Drawing for the job (mm, zero at the part's lowest x, y, z). Coordinates: 2 decimals unless noted, no trailing zeros. Loops run counter-clockwise (first coordinate to the right, second up) from the corner with the lowest first, then second, coordinate; pieces in that order, holes last. Notation, with made-up numbers: (-20.75, 20) - (14.25, 20) arc R25 ccw to (14.25, 40) - close; hole circle Ø8 at (-27, -25). An arc over 180 degrees is marked (long way). One line per item, written item: value.
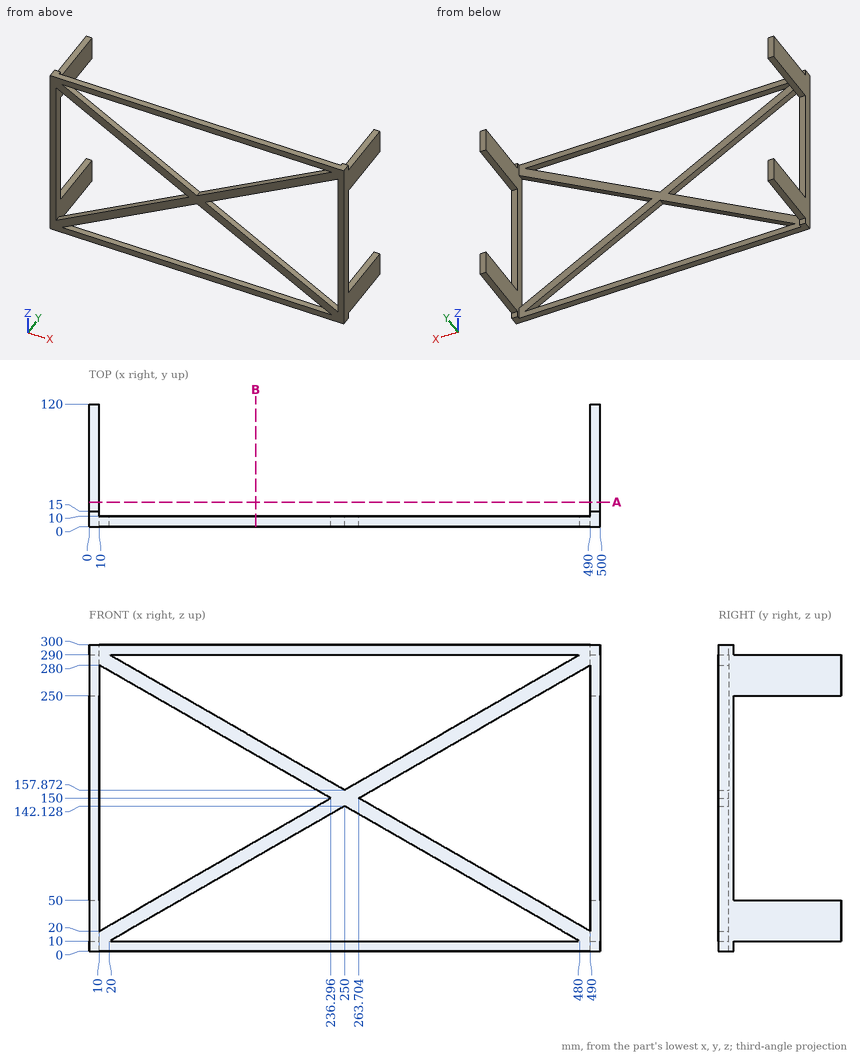
Item 1: Cut at B-B, the plane x = 163. Write the cut outline in (y, z), then the cut area to 3 significant figures.
Check result:
outline: (0, 0) - (10, 0) - (10, 10) - (0, 10) - close; (0, 92.15) - (10, 92.15) - (10, 107.89) - (0, 107.89) - close; (0, 192.11) - (10, 192.11) - (10, 207.85) - (0, 207.85) - close; (0, 290) - (10, 290) - (10, 300) - (0, 300) - close
area: 515 mm^2
Item 2: Probe probe 1 along X at (y, z) = (7, 129); probe 2 along X at (y, z) = (6, 217) (1 decimal); probe 3 along X at (y, z) = (63, 282). List the from-to ranges inside material, lowest first. Write a range as from..to.
Check result:
probe 1: x = 0..10, 199.74..227.15, 272.85..300.26, 490..500
probe 2: x = 0..10, 119.7..147.1, 352.9..380.3, 490..500
probe 3: x = 0..10, 490..500
Item 3: Cut at A-A, the plane y = 24. Write the cut outline in (x, z).
Check result:
outline: (0, 10) - (10, 10) - (10, 50) - (0, 50) - close; (0, 250) - (10, 250) - (10, 290) - (0, 290) - close; (490, 10) - (500, 10) - (500, 50) - (490, 50) - close; (490, 250) - (500, 250) - (500, 290) - (490, 290) - close
Item 4: Drop flat-ended pins along their axis: P1, Ø5, axis at x = 493.5, y = 83, coming from the -Z side; P2, Ø3, axis at x = 3.5, y = 45, coming from the +Z side; P3, Ø8, axis at x = 497, z = 3, coming from the +Y side. Give the stop position or say it passes through.
Check result:
P1: stops at z = 10
P2: stops at z = 290
P3: stops at y = 15
